Input: part model. Units: mm. Frame: model coordinates. Give positions to 0.01 mm unless a question says otherwise; leave off trailing zeros. Write each loop counter-clockwise with the first axis right and the second up, starting at its lowest first coordinate (ties: lowest second). Pieces come first, ordered by that corner, then holes.
```python
from build123d import *

# Parameters (mm, degrees)
ESBO_O1_W                  = 180
ESBO_O1_H                  = 120
RESSALTO_EXTRUS_O1_DEPTH   = 20
CORTE_EXTRUS_O1_DEPTH      = 152.327459504
CORTE_EXTRUS_O1_DEPTH_BACK = 152.327459504
ESBO_O2_R                  = 6


with BuildPart() as part:
    # Esboço1 → Ressalto-extrusão1 (new body)
    with BuildSketch(Plane.XY):
        with Locations((0, 60)):
            Rectangle(ESBO_O1_W, ESBO_O1_H)
    extrude(amount=RESSALTO_EXTRUS_O1_DEPTH)

    # Esboço2 → Corte-extrusão1 (cut, two sides: drawn at the far end of the back side and taken through both)
    with BuildSketch(Plane(origin=(0, 0, 0), x_dir=(-1, 0, 0), z_dir=(0, 0, -1)).offset(-CORTE_EXTRUS_O1_DEPTH_BACK)):
        with Locations((-50, 90)):
            Circle(ESBO_O2_R)
        with Locations((-50, 30)):
            Circle(ESBO_O2_R)
        with Locations((50, 30)):
            Circle(ESBO_O2_R)
        with Locations((50, 90)):
            Circle(ESBO_O2_R)
    extrude(amount=CORTE_EXTRUS_O1_DEPTH + CORTE_EXTRUS_O1_DEPTH_BACK, mode=Mode.SUBTRACT)


solid = part.part
```
Item 1: Section A-A (x = -50). Return loops of the section in (y, z), and give its area (3 significant figures).
Item 2: Section B-B (y = 90). Return loops of the section in (x, z).
Item 3: Section C-C (z = 17.5). Return loops of the section in (x, y).
Item 4: Pin query (flat end, axial travel): pin 1 (7 mm diameter, centred on x = 50, y = 30, fed in from +Z). Return the tip coordinate at first contact, or that it passes through.
Item 5: Ray query, line 1 (Y direction, x = 50, z = 15.75); line 2 (X direction, y = 30, z = 12.25); line 3 (Y direction, x = 51, z = 11.25). Return the intervals inside material, ascending.
Item 6: Mould query, pull axis Y, two halves, no side actions, for faces 1 (the cylindrical face through (-48.699, 24.143, 10.14)), 2 (the flat face through (-1, 61, 20)), 3 (the flat face through (-1, 120, 10)). Classes: +Y half, -Y half, draft (parallel to the pull), parting line (faces both ways), or undercut.
Solved:
1. outline: (0, 0) - (24, 0) - (24, 20) - (0, 20) - close; (36, 0) - (84, 0) - (84, 20) - (36, 20) - close; (96, 0) - (120, 0) - (120, 20) - (96, 20) - close
1. area: 1,920 mm2
2. outline: (-90, 0) - (-56, 0) - (-56, 20) - (-90, 20) - close; (-44, 0) - (44, 0) - (44, 20) - (-44, 20) - close; (56, 0) - (90, 0) - (90, 20) - (56, 20) - close
3. outline: (-90, 0) - (90, 0) - (90, 120) - (-90, 120) - close; hole circle Ø12 at (-50, 30); hole circle Ø12 at (-50, 90); hole circle Ø12 at (50, 30); hole circle Ø12 at (50, 90)
4. pin 1: passes through
5. line 1: y = 0 to 24, 36 to 84, 96 to 120
5. line 2: x = -90 to -56, -44 to 44, 56 to 90
5. line 3: y = 0 to 24.08, 35.92 to 84.08, 95.92 to 120
6. face 1: undercut
6. face 2: draft
6. face 3: +Y half
